Input: dimensioned drawing with shaded views. Units: mm. Origin: part minimum x, y, z. A direction names the side the tool comes from. Round coordinates to 2 decimals unless told otherwise and drop trailing zeros. Loops run counter-clockwise (first coordinate to the right, second up) from the corner with the lowest first, then second, coordinate; pieces in that order, holes last.
Item 1: Ray query, L1, parallel to Z at x = 0.85, y = 2; L2, parallel to Z at x = 3.4, y = 1.45; L3, parallel to X at y = 1.95, z = 12.5. Return the intervals inside material, ascending.
Item 2: Section query A-A on y = 2.5. Return loops of the section in (x, z), then the cut area to 3 significant figures.
Item 3: Access query for the marked faces 4 and 5. Directions: +Z, -Z, +X, -X, +Y, -Y. A direction counts if a zero-diameter tool reaches every point of the face in a straight line with its end or side. Return the directions, or none.
Item 4: Pull-direction query (Z, two-part tool) for the marked faces 1, 2 and 3; classes: released by +Z, released by -Z, zero draft, split by the parting line, or undercut.
Item 5: Section query D-D on x = 1.2. Return loops of the section in (y, z).
Item 6: First-contact query: P1, Ø1, axis at x = 1.5, y = 4, coming from the +Z side; P2, Ø1.5, axis at x = 3, z = 10, coming from the +Y side; P3, Ø1, axis at y = 1, z = 8.5, coming from the -X side. Flat tips, straight axial feed; report the tip coordinate or a pass-through.
Item 7: Section query C-C on z = 1.5. Return loops of the section in (x, y).
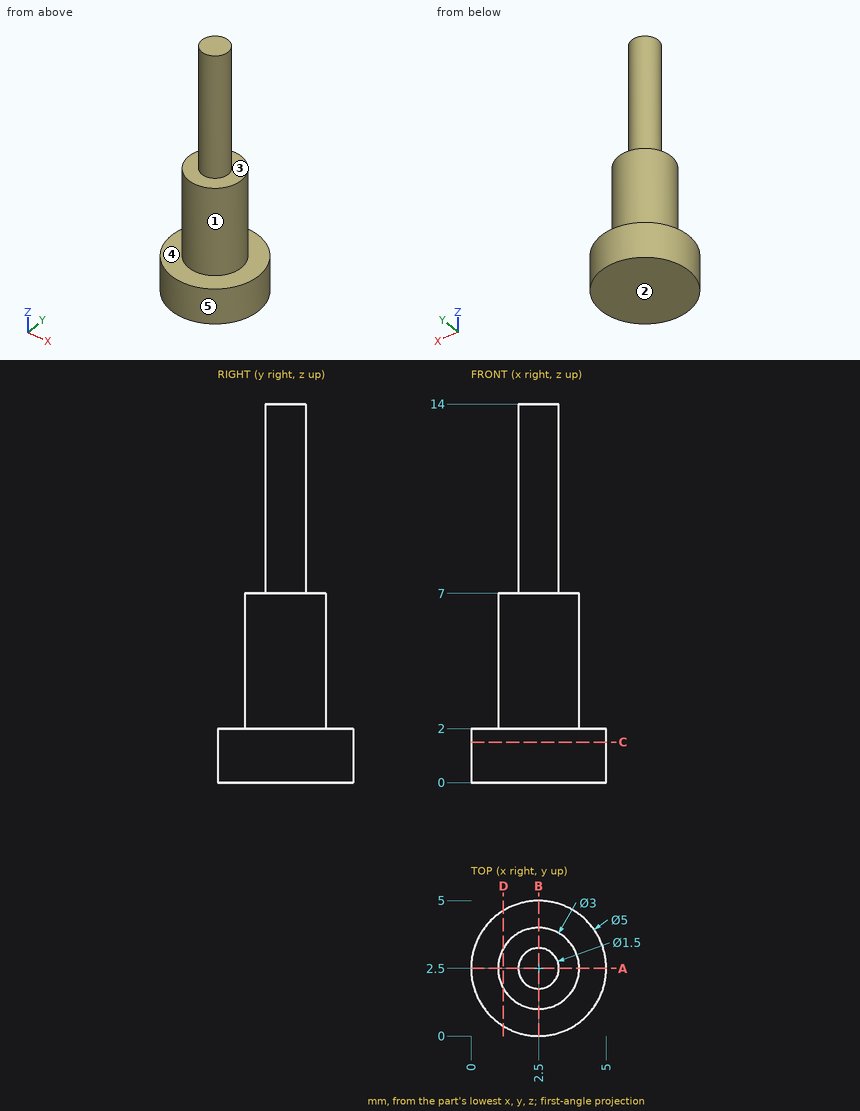
Data:
1. L1: z = 0 to 2
1. L2: z = 0 to 7
1. L3: x = 1.99 to 3.01
2. outline: (0, 0) - (5, 0) - (5, 2) - (4, 2) - (4, 7) - (3.25, 7) - (3.25, 14) - (1.75, 14) - (1.75, 7) - (1, 7) - (1, 2) - (0, 2) - close
2. area: 35.5 mm2
3. face 4: +Z
3. face 5: +Z, -Z
4. face 1: zero draft
4. face 2: released by -Z
4. face 3: released by +Z
5. outline: (0.36, 0) - (4.64, 0) - (4.64, 2) - (3.25, 2) - (3.25, 7) - (1.75, 7) - (1.75, 2) - (0.36, 2) - close
6. P1: stops at z = 7
6. P2: stops at y = 3.25
6. P3: passes through
7. outline: circle Ø5 at (2.5, 2.5)
